Geometry check sheet. Reference: the model listing, model coordinates, mm. Face numbers are marked on the shaded views. Coordinates: 2 decimals unless noted, no trailing zeros. Write each loop counter-clockwise with the first axis right and the second up, starting at its lowest first coordinate (ties: lowest second). Pieces come first, ordered by that corner, then holes. Notation, with made-up numbers: (-15.75, -12) -> (6.25, -12) arc R23 ccw to (6.25, 2) -> close; hole circle Ø6 at (48.25, 73.25). An arc over 180 degrees is marked (long way). Answer in a Markdown table with one row per item. Add a question column.
1. Mould release check, pull along Z, two halves, no side actions. Record for the marked faces 1, 2 and 3: pulls with the +Z half, pulls with the -Z half, needs draft (parallel to the pull), parting line crosses it, or undercut.
2. Cross-section at A-A on y = 13.5. Record the cut outline in (x, z), and give its area (3 significant figures).
3. Depth check by flat-ended pin: P1, Ø2, axis at x = -9, z = -0.5, coming from the -Y side; P2, Ø5, axis at x = -35.2, y = 0, coming from the +Z side; P3, Ø3.5, axis at x = -0.5, y = -0.5, coming from the -Z side. Enter the tip coordinate at first touch or a pass-through.
4. Cross-section at B-B on y = 0. Give the number of separate pieces and of enclosed holes in the cut face, and give its area (3 significant figures).
5. Cross-section at D-D on z = 31. Record the cut outline in (x, y).
6. Scan lines: L1, parallel to Z at x = 6.5, y = 1; L2, parallel to Y at x = 0, z = 15.5; L3, parallel to Z at x = 22.5, y = 4.5. Record each from-to range of solid material in increasing order. Write a range as from..to.
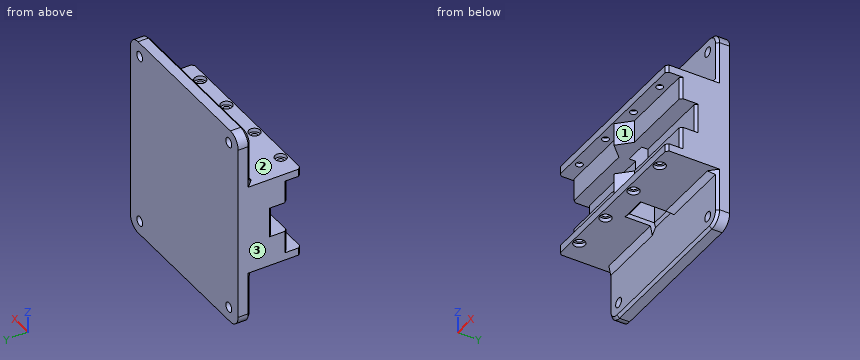
```python
from build123d import *

# Parameters (mm, degrees)
BOSS_EXTRUDE1_DEPTH        = 18
CROQUIS2_R                 = 1.35
CORTAR_EXTRUIR2_DEPTH      = 5
SKETCH3_R                  = 2.25
CUT_EXTRUDE1_DEPTH         = 1.5
CORTAR_EXTRUIR3_START      = 3
CORTAR_EXTRUIR3_DEPTH      = 17
CORTAR_EXTRUIR4_DEPTH      = 50.79015967
CORTAR_EXTRUIR4_DEPTH_BACK = 6
CROQUIS4_W                 = 70
CROQUIS4_H                 = 12
CORTAR_EXTRUIR11_DEPTH     = 60.498739482
CROQUIS6_W                 = 70
CROQUIS6_H                 = 80
CROQUIS6_R                 = 1.9
SALIENTE_EXTRUIR1_DEPTH    = 5
REDONDEO1_R                = 5
CHAFL_N1_SIZE              = 1
CHAFL_N2_SIZE              = 1
CHAFL_N3_SIZE              = 1
CHAFL_N5_SIZE              = 1
CHAFL_N6_SIZE              = 2


# Some blends are built 0.0001 mm under size
with BuildPart() as part:
    # Sketch1 → Boss-Extrude1 (new body)
    with BuildSketch(Plane.XY):
        Polygon((25.9, 17.3), (-9.1, 17.3), (-44.1, 17.3), (-44.1, -2.7), (-9.1, -2.7), (25.9, -2.7), (25.9, 2.5), align=None)
    boss_extrude1 = extrude(amount=BOSS_EXTRUDE1_DEPTH)

    # Croquis2 → Cortar-Extruir2 (cut)
    with BuildSketch(Plane.XY.offset(18)):
        Circle(CROQUIS2_R)
        with Locations((17, 0)):
            Circle(CROQUIS2_R)
        with Locations((-18.2, 0)):
            Circle(CROQUIS2_R)
        with Locations((-35.2, 0)):
            Circle(CROQUIS2_R)
    cortar_extruir2 = extrude(amount=-CORTAR_EXTRUIR2_DEPTH, mode=Mode.SUBTRACT)

    # Sketch3 → Cut-Extrude1 (cut)
    with BuildSketch(Plane.XY.offset(18)):
        Circle(SKETCH3_R)
        with Locations((17, 0)):
            Circle(SKETCH3_R)
        with Locations((-18.2, 0)):
            Circle(SKETCH3_R)
        with Locations((-35.2, 0)):
            Circle(SKETCH3_R)
    cut_extrude1 = extrude(amount=-CUT_EXTRUDE1_DEPTH, mode=Mode.SUBTRACT)

    # Croquis3 → Cortar-Extruir3 (cut)
    with BuildSketch(Plane(origin=(0, 0, 18), x_dir=(-1, 0, 0), z_dir=(0, 0, -1)).offset(CORTAR_EXTRUIR3_START)):
        Polygon((-25.9, -2.7), (-25.9, 2.8), (4.1, 2.8), (9.1, -2.2), (14.1, 2.8), (44.1, 2.8), (44.1, -2.7), align=None)
    cortar_extruir3 = extrude(amount=CORTAR_EXTRUIR3_DEPTH, mode=Mode.SUBTRACT)

    # Mirror1: Boss-Extrude1, Cortar-Extruir2, Cut-Extrude1, Cortar-Extruir3 across plane
    add(boss_extrude1.mirror(Plane(origin=(0, 0, 0), x_dir=(1, 0, 0), z_dir=(0, 0, -1))))
    add(cortar_extruir2.mirror(Plane(origin=(0, 0, 0), x_dir=(1, 0, 0), z_dir=(0, 0, -1))), mode=Mode.SUBTRACT)
    add(cut_extrude1.mirror(Plane(origin=(0, 0, 0), x_dir=(1, 0, 0), z_dir=(0, 0, -1))), mode=Mode.SUBTRACT)
    add(cortar_extruir3.mirror(Plane(origin=(0, 0, 0), x_dir=(1, 0, 0), z_dir=(0, 0, -1))), mode=Mode.SUBTRACT)

    # Croquis4 → Cortar-Extruir4 (cut, two sides: drawn at the far end of the back side and taken through both)
    with BuildSketch(Plane.XZ.offset(-2.8).offset(-CORTAR_EXTRUIR4_DEPTH_BACK)):
        with Locations((-9.1, 0)):
            Rectangle(CROQUIS4_W, CROQUIS4_H)
    extrude(amount=CORTAR_EXTRUIR4_DEPTH + CORTAR_EXTRUIR4_DEPTH_BACK, mode=Mode.SUBTRACT)

    # Croquis5 → Cortar-Extruir11 (cut, through all)
    with BuildSketch(Plane.XY.offset(18)):
        Polygon((-13.1, 10.671649133), (-13.1, 16.3), (-5.1, 16.3), (-5.1, 11.3), (-5.1, 6.3), (-13.1, 6.3), align=None)
    extrude(amount=-CORTAR_EXTRUIR11_DEPTH, mode=Mode.SUBTRACT)

    # Croquis6 → Saliente-Extruir1 (add)
    with BuildSketch(Plane(origin=(0, 17.3, 0), x_dir=(1, 0, 0), z_dir=(0, 1, 0))):
        with Locations((-9.1, 0)):
            Rectangle(CROQUIS6_W, CROQUIS6_H)
        with Locations(Location((-38.025442436, -34.47199994, 0), (0, 0, 180))):
            Circle(CROQUIS6_R, mode=Mode.SUBTRACT)
        with Locations((19.825442436, -34.47199994)):
            Circle(CROQUIS6_R, mode=Mode.SUBTRACT)
        with Locations(Location((19.825442436, 34.47199994, 0), (0, 0, 180))):
            Circle(CROQUIS6_R, mode=Mode.SUBTRACT)
        with Locations((-38.025442436, 34.47199994)):
            Circle(CROQUIS6_R, mode=Mode.SUBTRACT)
    extrude(amount=SALIENTE_EXTRUIR1_DEPTH)

    # Redondeo1
    redondeo1_edges = [part.edges().sort_by_distance(p)[0] for p in [
        (25.9, 19.8, 40),
        (25.9, 19.8, -40),
        (-44.1, 19.8, -40),
        (-44.1, 19.8, 40),
    ]]
    fillet(redondeo1_edges, radius=REDONDEO1_R)

    # Chaflán1
    chafl_n1_edges = [part.edges().sort_by_distance(p)[0] for p in [
        (-13.1, 11.3, 18),
        (-9.1, 6.3, 18),
        (-5.1, 11.3, 18),
        (-9.1, 16.3, 18),
    ]]
    chamfer(chafl_n1_edges, length=CHAFL_N1_SIZE - 0.0001)  # a hair under: the kernel refuses the full size

    # Chaflán2
    chafl_n2_edges = [part.edges().sort_by_distance(p)[0] for p in [
        (-9.1, 6.3, -18),
        (-13.1, 11.3, -18),
        (-5.1, 11.3, -18),
        (-9.1, 16.3, -18),
    ]]
    chamfer(chafl_n2_edges, length=CHAFL_N2_SIZE - 0.0001)  # a hair under: the kernel refuses the full size

    # Chaflán3
    chafl_n3_edges = [part.edges().sort_by_distance(p)[0] for p in [
        (25.9, 17.3, -26.5),
        (-44.1, 17.3, 26.5),
        (25.9, 17.3, 26.5),
        (-9.1, 17.3, 40),
        (-42.635533906, 17.3, 38.535533906),
        (24.435533906, 17.3, 38.535533906),
        (-44.1, 17.3, -26.5),
        (-9.1, 17.3, -40),
        (-42.635533906, 17.3, -38.535533906),
        (24.435533906, 17.3, -38.535533906),
    ]]
    chamfer(chafl_n3_edges, length=CHAFL_N3_SIZE)

    # Chaflán5
    chafl_n5_edges = [part.edges().sort_by_distance(p)[0] for p in [
        (25.9, -2.7, -16.5),
        (-44.1, -2.7, 16.5),
        (25.9, -2.7, 16.5),
        (25.9, 2.8, 10.5),
        (-44.1, 2.8, 10.5),
        (-44.1, 8.8, 0),
        (25.9, 8.8, 0),
        (-44.1, 2.8, -10.5),
        (25.9, 2.8, -10.5),
        (-44.1, -2.7, -16.5),
    ]]
    chamfer(chafl_n5_edges, length=CHAFL_N5_SIZE)

    # Chaflán6
    # the kernel refuses this chamfer: 2 mm, written as the material it adds along each edge
    with BuildSketch(Plane(origin=(-48.243365976, 17.3, 18), x_dir=(0, -0.9996219169112968, -0.027495876610585623), z_dir=(1, 0, 0))) as chafl_n6_piece_1_section:
        Polygon((CHAFL_N6_SIZE * 0.999621916911, -CHAFL_N6_SIZE * 0.0274958766106), (-CHAFL_N6_SIZE * 0.0274958766106, -CHAFL_N6_SIZE * 0.999621916911), (0, 0), align=None)
    chafl_n6_piece_1 = extrude(amount=78.286731952, mode=Mode.PRIVATE)
    chafl_n6_piece_1 = split(chafl_n6_piece_1, bisect_by=Plane(origin=(-21.681250309, 16.637349381, 25.581350309), z_dir=(-0.7071067811865476, 0, -0.7071067811865476)), keep=Keep.TOP, mode=Mode.PRIVATE)
    chafl_n6_piece_1 = split(chafl_n6_piece_1, bisect_by=Plane(origin=(-35.518649691, 9.718649691, 18.662650619), z_dir=(0.7071067811865476, 0.7071067811865476, 0)), keep=Keep.TOP, mode=Mode.PRIVATE)
    add(chafl_n6_piece_1)
    with BuildSketch(Plane(origin=(-48.243365976, 17.3, 18), x_dir=(0, -0.9996219169112968, -0.027495876610585623), z_dir=(1, 0, 0))) as chafl_n6_piece_2_section:
        Polygon((CHAFL_N6_SIZE * 0.999621916911, -CHAFL_N6_SIZE * 0.0274958766106), (-CHAFL_N6_SIZE * 0.0274958766106, -CHAFL_N6_SIZE * 0.999621916911), (0, 0), align=None)
    chafl_n6_piece_2 = extrude(amount=78.286731952, mode=Mode.PRIVATE)
    chafl_n6_piece_2 = split(chafl_n6_piece_2, bisect_by=Plane(origin=(17.318649691, 9.718649691, 18.662650619), z_dir=(-0.7071067811865476, 0.7071067811865476, 0)), keep=Keep.TOP, mode=Mode.PRIVATE)
    chafl_n6_piece_2 = split(chafl_n6_piece_2, bisect_by=Plane(origin=(3.481250309, 16.637349381, 25.581350309), z_dir=(0.7071067811865476, 0, -0.7071067811865476)), keep=Keep.TOP, mode=Mode.PRIVATE)
    add(chafl_n6_piece_2)
    with BuildSketch(Plane(origin=(-48.243365976, 17.3, -18), x_dir=(0, -0.9996219169112968, 0.027495876610585623), z_dir=(1, 0, 0))) as chafl_n6_piece_3_section:
        Polygon((CHAFL_N6_SIZE * 0.999621916911, CHAFL_N6_SIZE * 0.0274958766106), (-CHAFL_N6_SIZE * 0.0274958766106, CHAFL_N6_SIZE * 0.999621916911), (0, 0), align=None)
    chafl_n6_piece_3 = extrude(amount=78.286731952, mode=Mode.PRIVATE)
    chafl_n6_piece_3 = split(chafl_n6_piece_3, bisect_by=Plane(origin=(-21.681250309, 16.637349381, -25.581350309), z_dir=(-0.7071067811865476, 0, 0.7071067811865476)), keep=Keep.TOP, mode=Mode.PRIVATE)
    chafl_n6_piece_3 = split(chafl_n6_piece_3, bisect_by=Plane(origin=(-35.518649691, 9.718649691, -18.662650619), z_dir=(0.7071067811865476, 0.7071067811865476, 0)), keep=Keep.TOP, mode=Mode.PRIVATE)
    add(chafl_n6_piece_3)
    with BuildSketch(Plane(origin=(-48.243365976, 17.3, -18), x_dir=(0, -0.9996219169112968, 0.027495876610585623), z_dir=(1, 0, 0))) as chafl_n6_piece_4_section:
        Polygon((CHAFL_N6_SIZE * 0.999621916911, CHAFL_N6_SIZE * 0.0274958766106), (-CHAFL_N6_SIZE * 0.0274958766106, CHAFL_N6_SIZE * 0.999621916911), (0, 0), align=None)
    chafl_n6_piece_4 = extrude(amount=78.286731952, mode=Mode.PRIVATE)
    chafl_n6_piece_4 = split(chafl_n6_piece_4, bisect_by=Plane(origin=(3.481250309, 16.637349381, -25.581350309), z_dir=(0.7071067811865476, 0, 0.7071067811865476)), keep=Keep.TOP, mode=Mode.PRIVATE)
    chafl_n6_piece_4 = split(chafl_n6_piece_4, bisect_by=Plane(origin=(17.318649691, 9.718649691, -18.662650619), z_dir=(-0.7071067811865476, 0.7071067811865476, 0)), keep=Keep.TOP, mode=Mode.PRIVATE)
    add(chafl_n6_piece_4)


solid = part.part
```
Results found:
| question | item | result |
|---|---|---|
| 1 | face 1 | undercut |
| 1 | face 2 | pulls with the +Z half |
| 1 | face 3 | needs draft |
| 2 | outline | (-44.1, -18) -> (-14.1, -18) -> (-13.1, -17) -> (-13.1, 17) -> (-14.1, 18) -> (-44.1, 18) -> close; (-5.1, -17) -> (-4.1, -18) -> (25.9, -18) -> (25.9, 18) -> (-4.1, 18) -> (-5.1, 17) -> close |
| 2 | area | 2,230 mm^2 |
| 3 | P1 | stops at y = 16.3 |
| 3 | P2 | stops at z = 18 |
| 3 | P3 | stops at z = -18 |
| 4 | separate pieces | 10 |
| 4 | enclosed holes | 0 |
| 4 | area | 413 mm^2 |
| 5 | outline | (-44.1, 18.3) -> (-43.1, 17.3) -> (24.9, 17.3) -> (25.9, 18.3) -> (25.9, 22.3) -> (-44.1, 22.3) -> close |
| 6 | L1 | z = -18..-15, 15..18 |
| 6 | L2 | y = -2.7..-1.35, 1.35..22.3 |
| 6 | L3 | z = -18..-6, 6..18 |
